from build123d import *

# Parameters (mm, degrees)
SKETCH2_R          = 3
CUT_EXTRUDE1_DEPTH = 60.674115125


with BuildPart() as part:
    # Sketch1 → Revolve1 (revolve)
    with BuildSketch(Plane.XY, mode=Mode.PRIVATE) as revolve1_sk:
        with BuildLine():
            Line((27, 4), (27, 2.5))
            Line((27, 2.5), (20, 2.5))
            Line((20, 2.5), (0.5, 2.5))
            Line((0.5, 2.5), (0.5, 30.5))
            ThreePointArc((0.5, 30.5), (10, 40), (19.5, 30.5))
            Line((19.5, 30.5), (19.5, 6.5))
            Line((19.5, 6.5), (20, 6.5))
            Line((20, 6.5), (20, 4))
            Line((20, 4), (27, 4))
        make_face()
    revolve(revolve1_sk.sketch.rotate(Axis((0, 0, 0), (1, 0, 0)), 90), axis=Axis((0, 0, 0), (1, 0, 0)))

    # Sketch2 → Cut-Extrude1 (cut, through all)
    with BuildSketch(Plane(origin=(19.5, 0, 0), x_dir=(0, 0, -1), z_dir=(1, 0, 0))):
        with Locations((-15.5, 15.5)):
            Circle(SKETCH2_R)
        with Locations((15.5, 15.5)):
            Circle(SKETCH2_R)
        with Locations((15.5, -15.5)):
            Circle(SKETCH2_R)
        with Locations((-15.5, -15.5)):
            Circle(SKETCH2_R)
    extrude(amount=-CUT_EXTRUDE1_DEPTH, mode=Mode.SUBTRACT)


solid = part.part
Build history of the part. All positions in model axes, mm. A direction names the side the tool comes from. Round coordinates to 2 decimals unless told otherwise and drop trailing zeros. Loops run counter-clockwise (first coordinate to the right, second up) from the corner with the lowest first, then second, coordinate; pieces in that order, holes last. Notation, with made-up numbers: (40, 38.5) -> (62, 38.5) arc R11 cw to (62, 47.5) -> close; hole circle Ø7 at (14.5, 53). An arc over 180 degrees is marked (long way). Answer in a Markdown table with one row per item.
Item 1: Drill centre lines: L1, parallel to Y at x = 12.75, z = 15.5; L2, parallel to Y at x = 7.5, z = -14.5; L3, parallel to Z at x = 3, y = 15. Where is each one in solid material? Low to high. Write a range as [from, to].
Answers below:
| item | result |
|---|---|
| L1 | y = [-36.43, -18.5], [-12.5, 12.5], [18.5, 36.43] |
| L2 | y = [-36.92, -18.33], [-12.67, 12.67], [18.33, 36.92] |
| L3 | z = [-33.74, -18.46], [-12.54, 12.54], [18.46, 33.74] |
Item 2: Pin check, flat tips, straight feed: pin 1 (8 mm diameter, centred on y = 15.5, z = 15.5, fed in from +X); pin 2 (5 mm diameter, centred on y = -15.5, z = -15.5, fed in from +X); pin 3 (12 mm diameter, centred on y = 2.5, z = -10.5, fed in from +X); pin 4 (4 mm diameter, centred on x = 9, z = 7.5, fed in from +Y). Stop position of each tip, or through.
Answers below:
| item | result |
|---|---|
| pin 1 | stops at x = 19.5 |
| pin 2 | passes through |
| pin 3 | stops at x = 20 |
| pin 4 | stops at y = 39.6 |
Item 3: Mould opens along Z. For faces 1 (the cylindrical face through (23.549, 3.905, -0.867)), 2 (the flat face through (27, -2, 2)), 3 (the cylindrical face through (13.6, -0.1, -2.5)) say: +Z half, -Z half, draft (parallel to the pull), parting line (faces both ways), or undercut.
Answers below:
| item | result |
|---|---|
| face 1 | parting line |
| face 2 | draft |
| face 3 | undercut |
Item 4: Which spindle directions (+Z, -Z, +X, -X, +Y, -Y) get a long thin tool onto all of the face, cutting with end or side? Do faces 4 (the cylindrical face through (10.1, 13.7, -13.1)), 5 (the flat face through (20, -3, 3)). Say none if no direction does.
Answers below:
| item | result |
|---|---|
| face 4 | +X, -X |
| face 5 | +X |
Item 5: Saw through at C-C (x = 14). Write the cut outline in (y, z), and give its area (3 significant figures).
Answers below:
| item | result |
|---|---|
| outline | circle Ø78.23 at (0, 0); hole circle Ø6 at (-15.5, -15.5); hole circle Ø6 at (-15.5, 15.5); hole circle Ø5 at (0, 0); hole circle Ø6 at (15.5, -15.5); hole circle Ø6 at (15.5, 15.5) |
| area | 4,670 mm² |
Item 6: Saw through at D-D (x = 23.75). Write the cut outline in (y, z), and give its area (3 significant figures).
Answers below:
| item | result |
|---|---|
| outline | circle Ø8 at (0, 0); hole circle Ø5 at (0, 0) |
| area | 30.6 mm² |
Item 7: Saw through at A-A (z = 0). Write the cut outline in (x, y), and give its area (3 significant figures).
Answers below:
| item | result |
|---|---|
| outline | (0.5, -30.5) arc R9.5 ccw to (19.5, -30.5) -> (19.5, -6.5) -> (20, -6.5) -> (20, -4) -> (27, -4) -> (27, -2.5) -> (0.5, -2.5) -> close; (0.5, 2.5) -> (27, 2.5) -> (27, 4) -> (20, 4) -> (20, 6.5) -> (19.5, 6.5) -> (19.5, 30.5) arc R9.5 ccw to (0.5, 30.5) -> close |
| area | 1,370 mm² |
